Could you check a few things on this model? Use its own coordinates, in mm. A direction names the side the tool comes from. Coordinates: 2 decimals unless noted, no trailing zeros. Loops run counter-clockwise (first coordinate to the right, second up) from the corner with the lowest first, then second, coordinate; pieces in that order, holes last. Notation, with made-up numbers: (75.25, 87.5) - (109.25, 87.5) arc R26 ccw to (109.25, 121.5) - close; hole circle Ø11 at (83.25, 35.25). An arc over 180 degrees is marked (long way). Put each result on its own line as item: value. Start each with the question number.
```python
from build123d import *

# Parameters (mm, degrees)
BOSS_EXTRUDE1_DEPTH    = 1.5875
F_10_CLEARANCE_HOLE1_D = 4.9784
SKETCH5_R              = 14.057169334
CUT_EXTRUDE1_DEPTH     = 2.54
F_10_CLEARANCE_HOLE2_D = 4.9784


with BuildPart() as part:
    # Sketch2 → Boss-Extrude1 (new body)
    with BuildSketch(Plane(origin=(0, 0, 189.78999271), x_dir=(-1, 0, 0), z_dir=(0, 0, -1))):
        Polygon((57.864732818, -87.431436787), (84.784631441, -130.512280072), (98.247394968, -122.099811752), (141.333866252, -191.052579482), (184.414709536, -164.132680859), (114.40833963, -52.099069844), align=None)
    extrude(amount=BOSS_EXTRUDE1_DEPTH)

    # #10 Clearance Hole1 (through all)
    with Locations(Plane(origin=(0, 0, 188.20249271), x_dir=(-1, 0, 0), z_dir=(0, 0, -1))):
        with Locations((106.997487706, -124.119929835), (86.804749524, -121.762187333), (112.388221547, -60.849162582), (132.578145514, -93.159795046), (139.30812017, -103.930005867), (172.792086333, -157.515553088), (140.48145387, -177.705477055)):
            Hole(F_10_CLEARANCE_HOLE1_D / 2)

    # Sketch5 → Cut-Extrude1 (cut)
    with BuildSketch(Plane.XY.offset(189.78999271)):
        with Locations((-92.865103341, -95.511909387)):
            Circle(SKETCH5_R)
    extrude(amount=-CUT_EXTRUDE1_DEPTH, mode=Mode.SUBTRACT)

    # #10 Clearance Hole2 (through all)
    with Locations(Plane.XY.offset(189.78999271)):
        with Locations((-66.614825557, -89.451554869)):
            Hole(F_10_CLEARANCE_HOLE2_D / 2)


solid = part.part
```
(1) I want a section at D-D on x = -76. List the corners of the cut face in (y, z) for me.
(2) If we mould it in two halves opening along Y, with no side actions, what happens to faces 1 (the cylindrical face through (-87.3, -124.2, 189)), 2 (the flat face through (-162.573, -177.781, 189.007)), 3 (the flat face through (-149.9, -108.9, 189))? For each: pulls with the +Y half, pulls with the -Y half, needs draft (parallel to the pull), parting line crosses it, or undercut.
(3) I need wall thicknesses on L1, parallel to X at y = -124.5, z = 189.3; L2, parallel to X at y = -159, z = 189; L3, parallel to X at y = -94.5, z = 188.8. Which ranges of each line are inside material? Lowest first, please. Write a range as [from, to].
(4) I want a section at C-C on y = -172. List the corners of the cut face in (x, z) for me, and give its area (3 significant figures).
(5) For pin 1 Ø12 at (x, y) = (-97, -137) entering from +Z, with a flat end and sliding along its axis, tell me the tip position at first contact or that it passes through.
(6) Which directions (+Z, -Z, +X, -X, +Y, -Y) give clear straight access to the entire face, cutting with the end or side of a thin tool? Please do faces 4 (the flat face through (-120, -121, 189.79)), 5 (the flat face through (-91.422, -126.365, 189.007)).
(7) I want a section at B-B on z = 188.55. Count the separate pieces of the cut face and the enclosed holes in it, and give its area (3 significant figures).
(8) I want a section at A-A on x = -173.5. List the corners of the cut face in (y, z) for me.
Answer sheet:
1. outline: (-116.45, 188.2) - (-76.1, 188.2) - (-76.1, 189.79) - (-116.45, 189.79) - close
2. face 1: undercut
2. face 2: pulls with the -Y half
2. face 3: pulls with the +Y half
3. L1: x = [-159.65, -109.46], [-104.54, -99.75], [-94.41, -81.03]
3. L2: x = [-181.21, -174.79], [-170.79, -121.31]
3. L3: x = [-140.9, -134.68], [-130.48, -106.89], [-78.84, -62.28]
4. outline: (-171.82, 188.2) - (-129.43, 188.2) - (-129.43, 189.79) - (-171.82, 189.79) - close
4. area: 67.3 mm^2
5. pin 1: passes through
6. face 4: +Z, +X, -X, +Y, -Y
6. face 5: +Z, -Z, -Y
7. separate pieces: 1
7. enclosed holes: 9
7. area: 6,740 mm^2
8. outline: (-170.95, 188.2) - (-159.9, 188.2) - (-159.9, 189.79) - (-170.95, 189.79) - close; (-155.13, 188.2) - (-146.67, 188.2) - (-146.67, 189.79) - (-155.13, 189.79) - close
